```python
from build123d import *

# Parameters (mm, degrees)
SKETCH_1_R          = 40
EXTRUDE_1_DEPTH     = 11.8
SKETCH_2_R          = 2.15
SKETCH_2_R_2        = 1.75
CUT_EXTRUDE_1_DEPTH = 58.786157512
SKETCH_3_R          = 3.025
SKETCH_3_R_2        = 15.6
CUT_EXTRUDE_2_DEPTH = 58.786157512
SKETCH_5_R          = 2.9
SKETCH_5_R_2        = 3.5
CUT_EXTRUDE_4_DEPTH = 4


with BuildPart() as part:
    # 草图1 → 凸台-拉伸1 (new body)
    with BuildSketch(Plane.XY):
        Circle(SKETCH_1_R)
    extrude(amount=EXTRUDE_1_DEPTH)

    # 草图2 → 切除-拉伸1 (cut, through all)
    with BuildSketch(Plane(origin=(0, 0, 0), x_dir=(-1, 0, 0), z_dir=(0, 0, -1))):
        with Locations((-32.730643847, 10.1245665)):
            Circle(SKETCH_2_R)
        with Locations(Location((-32.730643847, -9.8754335, 0), (0, 0, 180))):
            Circle(SKETCH_2_R)
        with Locations((32.269356153, -9.8754335)):
            Circle(SKETCH_2_R)
        with Locations(Location((32.269356153, 10.1245665, 0), (0, 0, 180))):
            Circle(SKETCH_2_R)
        with Locations((-9.290643847, 33.9345665)):
            Circle(SKETCH_2_R_2)
        with Locations(Location((8.829356153, 33.9345665, 0), (0, 0, 180))):
            Circle(SKETCH_2_R_2)
        with Locations((8.829356153, -33.6854335)):
            Circle(SKETCH_2_R_2)
        with Locations(Location((-9.290643847, -33.6854335, 0), (0, 0, 180))):
            Circle(SKETCH_2_R_2)
    extrude(amount=-CUT_EXTRUDE_1_DEPTH, mode=Mode.SUBTRACT)

    # 草图3 → 切除-拉伸2 (cut, through all)
    with BuildSketch(Plane(origin=(0, 0, 0), x_dir=(-1, 0, 0), z_dir=(0, 0, -1))):
        with Locations((0, 31.5)):
            Circle(SKETCH_3_R)
        with Locations((27.279800219, 15.75)):
            Circle(SKETCH_3_R)
        with Locations((27.279800219, -15.75)):
            Circle(SKETCH_3_R)
        with Locations((0, -31.5)):
            Circle(SKETCH_3_R)
        with Locations((-27.279800219, -15.75)):
            Circle(SKETCH_3_R)
        with Locations((-27.279800219, 15.75)):
            Circle(SKETCH_3_R)
        Circle(SKETCH_3_R_2)
    extrude(amount=-CUT_EXTRUDE_2_DEPTH, mode=Mode.SUBTRACT)

    # 草图5 → 切除-拉伸4 (cut)
    with BuildSketch(Plane.XY.offset(11.8)):
        with Locations((-8.829356153, -33.6854335)):
            Circle(SKETCH_5_R)
        with Locations((-8.829356153, 33.9345665)):
            Circle(SKETCH_5_R)
        with Locations((-32.269356153, 10.1245665)):
            Circle(SKETCH_5_R_2)
        with Locations((-32.269356153, -9.8754335)):
            Circle(SKETCH_5_R_2)
        with Locations((9.290643847, 33.9345665)):
            Circle(SKETCH_5_R)
        with Locations((32.730643847, 10.1245665)):
            Circle(SKETCH_5_R_2)
        with Locations((32.730643847, -9.8754335)):
            Circle(SKETCH_5_R_2)
        with Locations((9.290643847, -33.6854335)):
            Circle(SKETCH_5_R)
    extrude(amount=-CUT_EXTRUDE_4_DEPTH, mode=Mode.SUBTRACT)


solid = part.part
```
Input: part model. Units: mm. Frame: model coordinates. A direction names the side the tool comes from. Give positions to 0.01 mm unless a question says otherwise; leave off trailing zeros. Loops run counter-clockwise (first coordinate to the right, second up) from the corner with the lowest first, then second, coordinate; pieces in that order, holes last.
1) Section query A-A on y = 0. Return the cut outline in (x, z), and give its area (3 significant figures).
A:
outline: (-40, 0) - (-15.6, 0) - (-15.6, 11.8) - (-40, 11.8) - close; (15.6, 0) - (40, 0) - (40, 11.8) - (15.6, 11.8) - close
area: 576 mm2
2) Mould query, pull axis Y, two halves, no side actions, for faces 3 (the cylindrical face through (0.656, -34.453, 5.817)), 4 (the flat face through (17, 1, 0)). Classes: released by +Y, released by -Y, zero draft, split by the parting line, or undercut.
A:
face 3: undercut
face 4: zero draft
3) Section query B-B on x = 2. Return the cut outline in (y, z), and give its area (3 significant figures).
A:
outline: (-39.95, 0) - (-33.77, 0) - (-33.77, 11.8) - (-39.95, 11.8) - close; (-29.23, 0) - (-15.47, 0) - (-15.47, 11.8) - (-29.23, 11.8) - close; (15.47, 0) - (29.23, 0) - (29.23, 11.8) - (15.47, 11.8) - close; (33.77, 0) - (39.95, 0) - (39.95, 11.8) - (33.77, 11.8) - close
area: 471 mm2
4) Line query: L1, parallel to Y at x = 34, z = 1.25; L2, parallel to Y at x = 30, z = 1.5; L3, parallel to X at y = 9, z = 0.5. Output: solid intervals per line, ascending.
A:
L1: y = -21.07 to -11.61, -8.14 to 8.39, 11.86 to 21.07
L2: y = -26.46 to -17.07, -14.43 to 14.43, 17.07 to 26.46
L3: x = -38.97 to -34.1, -30.44 to -12.74, 12.74 to 30.9, 34.56 to 38.97
5) Contact query for flat-ended pins moving along their axis: pin 1 (2 mm diameter, centred on y = 3.5, z = 7, fed in from -X); pin 2 (5 mm diameter, centred on x = 32.73, y = -9.88, fed in from +Z); pin 3 (1 mm diameter, centred on x = -4.5, z = 3.5, fed in from +Y). Output: stop coordinate, or through.
A:
pin 1: stops at x = -39.92
pin 2: stops at z = 7.8
pin 3: stops at y = 39.8
6) Section query D-D on x = -26.5. Return the cut outline in (y, z), and give its area (3 significant figures).
A:
outline: (-29.96, 0) - (-18.67, 0) - (-18.67, 11.8) - (-29.96, 11.8) - close; (-12.83, 0) - (12.83, 0) - (12.83, 11.8) - (-12.83, 11.8) - close; (18.67, 0) - (29.96, 0) - (29.96, 11.8) - (18.67, 11.8) - close
area: 569 mm2
7) Section query C-C on z = 4.25. Count the separate pieces of the cut face and the enclosed holes in it, and give its area (3 significant figures).
A:
separate pieces: 1
enclosed holes: 15
area: 3,990 mm2
8) Reachability of faces 1 (the cylindrical face through (12.057, -32.814, 9.828)), 2 (the cylindrical face through (8.911, -31.977, 3.845)) from +Z, -Z, +X, -X, +Y, -Y: full face, straight path, thin tool, end or side. Return the list, or none.
A:
face 1: +Z
face 2: +Z, -Z
